The figure shows three views and two pictorial views of one solid part (mm, origin at its lowest corner). Answer the questions. Coordinates: 2 decimals unless noted, no trailing zeros. Order: outer loops, then holes, each group sorted by start corner. A loop starts at its lowest first (then second) coordinate and runs counter-clockwise, first axis right, second up. Notation, with made-up numbers: (62.5, 79.5) -> (90.5, 79.5) arc R30 ccw to (90.5, 116.5) -> close; hole circle Ø3 at (-34, -30). An arc over 180 degrees is marked (long way). Write item = value, one per line.
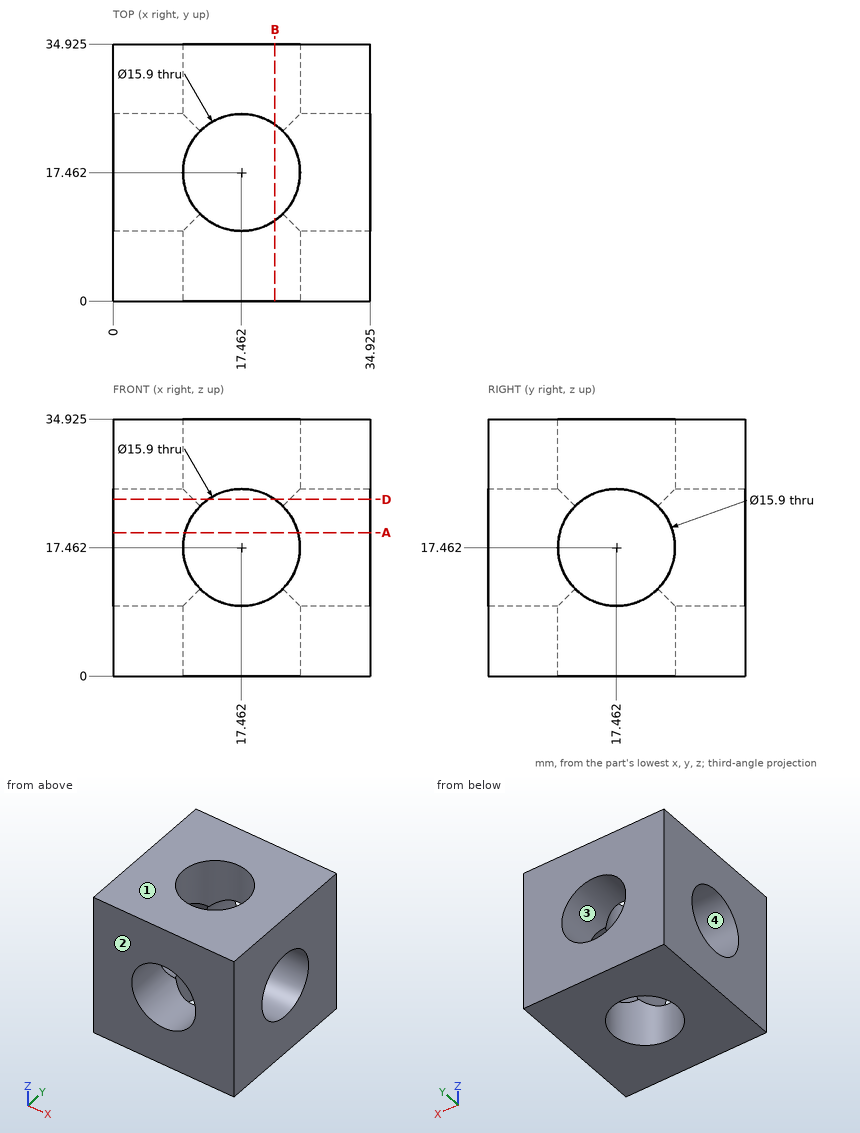
Q1. Section D-D, the plane z = 24 is taken. Give the number of separate pieces and of enclosed holes in the cut face.
The answers:
separate_pieces = 4
enclosed_holes = 0
Q2. This flat-tipped pin is pushed along its axis until it touches: pin 1 Ø18.5 at (x, z) = (17.46, 17.46) entering from -Y. Where does it stop, or does it pass through?
The answers:
pin_1 = 0
Q3. Section A-A, the plane z = 19.5 is taken. Give the vertices of the cut face in (x, y) (1 decimal).
The answers:
outline = (0, 0) -> (9.8, 0) -> (9.8, 9.8) -> (0, 9.8) -> close; (0, 25.1) -> (9.8, 25.1) -> (9.8, 34.9) -> (0, 34.9) -> close; (25.1, 0) -> (34.9, 0) -> (34.9, 9.8) -> (25.1, 9.8) -> close; (25.1, 25.1) -> (34.9, 25.1) -> (34.9, 34.9) -> (25.1, 34.9) -> close
Q4. Find the intervals of material crossed by line 1 along Y through (x, z) = (6, 17.5) (1 decimal); line 2 along X through (y, z) = (24, 26.5) (1 decimal), in increasing order.
The answers:
line_1 = 0 to 9.5, 25.4 to 34.9
line_2 = 0 to 12.9, 22 to 34.9
Q5. The mould has two halves that part along Z. Classify the marked faces 1, 2, 3 and 4: released by +Z, released by -Z, zero draft, split by the parting line, or undercut.
The answers:
face_1 = released by +Z
face_2 = zero draft
face_3 = undercut
face_4 = undercut
Q6. Section B-B, the plane x = 22 is taken. Give the vertices of the cut face in (y, z) (1 decimal), plus the area to 3 significant figures.
The answers:
outline = (0, 0) -> (10.9, 0) -> (10.9, 10.9) -> (0, 10.9) -> close; (0, 24) -> (10.9, 24) -> (10.9, 34.9) -> (0, 34.9) -> close; (24, 0) -> (34.9, 0) -> (34.9, 10.9) -> (24, 10.9) -> close; (24, 24) -> (34.9, 24) -> (34.9, 34.9) -> (24, 34.9) -> close
area = 478 mm2
